Autodesk Inventor part; units mm, degrees
ref_plane "Start plane" through (0, 0, 0) normal (0, 0, 1) x (1, 0, 0)
ref_plane "End plane" through (0, 0, 1500) normal (0, 0, 1) x (1, 0, 0)
ref_plane "YZ Plane" through (0, 0, 0) normal (1, 0, 0) x (0, 1, 0)
ref_plane "Start plane" through (0, 0, 0) normal (0, 0, 1) x (1, 0, 0)
ref_plane "End plane" through (0, 0, 1500) normal (0, 0, 1) x (1, 0, 0)
sketch "Sketch" plane through (0, 0, 0) normal (0, 0, 1) x (1, 0, 0)
  line L0 (-36.5, -70) -> (-36.5, -63.1)
  line L1 (-36.5, -63.1) -> (-9.35, -63.1)
  line L2 (-2.35, -56.1) -> (-2.35, 0)
  line L3 (-2.35, 0) -> (0, 0) construction
  line L4 (0, 0) -> (0, -70) construction
  line L5 (0, -70) -> (-36.5, -70)
  line L6 (-60, 0) -> (80, 0) construction
  line L7 (0, -60) -> (0, 80) construction
  line L8 (36.5, -70) -> (36.5, -63.1)
  line L9 (36.5, -63.1) -> (9.35, -63.1)
  line L10 (2.35, -56.1) -> (2.35, 0)
  line L11 (2.35, 0) -> (0, 0) construction
  line L12 (0, -70) -> (36.5, -70)
  line L13 (-36.5, 70) -> (-36.5, 63.1)
  line L14 (-36.5, 63.1) -> (-9.35, 63.1)
  line L15 (-2.35, 56.1) -> (-2.35, 0)
  line L16 (0, 70) -> (-36.5, 70)
  line L17 (36.5, 70) -> (36.5, 63.1)
  line L18 (36.5, 63.1) -> (9.35, 63.1)
  line L19 (0, 70) -> (36.5, 70)
  line L20 (2.35, 56.1) -> (2.35, 0)
  arc A0 (-2.35, 56.1) -> (-9.35, 63.1) centre (-9.35, 56.1) ccw
  arc A1 (9.35, 63.1) -> (2.35, 56.1) centre (9.35, 56.1) ccw
  arc A2 (2.35, -56.1) -> (9.35, -63.1) centre (9.35, -56.1) ccw
  arc A3 (-9.35, -63.1) -> (-2.35, -56.1) centre (-9.35, -56.1) ccw
  line L21 (0, 108) -> (0, -88) construction
  line L22 (-88, 0) -> (108, 0) construction
  point P0 (-2.35, -63.1)
  point P1 (2.35, -63.1)
  point P2 (-2.35, 63.1)
  point P3 (2.35, 63.1)
  dimension "d1" = 70
  dimension "d2" = 6.9
  dimension "d3" = 36.5
  dimension "d4" = 2.35
  dimension "d10" = 7
extrude "Body" add sketch "Sketch" along normal up to surface (1500 mm away) from surface at 0
sketch "Sketch4" plane through (0, 0, 0) normal (0, 0, 1) x (1, 0, 0)
  line L0 (0, 0) -> (10, 0)
ref_plane "Work Plane3" through (0, 0, 0) normal (0, -1, 0) x (1, 0, 0)
sketch "Sketch5" plane through (0, 0, 0) normal (0, -1, 0) x (1, 0, 0)
  line L0 (-2, 0) -> (12, 0)
  line L1 (-2, 1500) -> (12, 1500)
  dimension "d14" = 1500
equation "\"d1\" = 0.5 * G_H"
equation "\"d2\" = G_T1"
equation "\"d3\" = 0.5 * G_W"
equation "\"d4\" = 0.5 * G_T"
equation "\"d10\" = G_IR"
equation "\"d5\" = G_L"
equation "\"G_W\" = 73"
equation "\"G_T\" = 4.7"
equation "\"G_T1\" = 6.9"
equation "\"G_IR\" = 7"
equation "\"G_L\" = d14"
equation "\"G_OFFSET_START\" = 0"
equation "\"G_OFFSET_END\" = 0"
properties part number "PN-91/H-93419 - IPE140 - 1500" material "Steel, Mild"
Input: part model. Units: mm. Frame: model coordinates. A direction names the side the tool comes from. Coordinates: 2 decimals unless noted, no trailing zeros. Write each loop counter-clockwise with the first axis right and the second up, starting at its lowest first coordinate (ties: lowest second). Pieces come first, ordered by that corner, then holes. Notation, with made-up numbers: M -24.75,56 L -2.75,56 A20 ccw -2.75,80 Z; hole C -36,38 d5. An arc over 180 degrees is marked long. Answer as a JSON object with one key per item and string values. Group by question number.
(1) Ray query, line 1 along Y through (x, z) = (-28, 393); line 2 along X through (y, z) = (-6.5, 1286.5); line 3 along Y through (x, z) = (3, 564). Return the intervals inside material, ascending. Write a range as [from, to].
(2) Contact query for a flat-ended pin moving along its axis: P1, Ø3, axis at y = 23, z = 1046.5, coming from the -X side. Output: stop coordinate, or through.
(3) Set-up query: faces 1 (the face through (1, -70, 740)), 2 (the face through (2.35, 1, 740)), 3 (the face through (-2.35, 1, 740)). Return all of +Z, -Z, +X, -X, +Y, -Y with unobstructed straight access to the full face (end or side cutting, diameter ignored); none if empty.
(4) Section A-A on x = -21. Output: boundary loops of the cut face in (y, z).
(5) Section B-B on z = 730.5. Output: boundary loops of the cut face in (x, y), plus the area to 3 significant figures.
(6) Section C-C on y = -29. Output: boundary loops of the cut face in (x, z), plus the area to 3 significant figures.
Result set:
{
 "1": {"line 1": "y = [-70, -63.1], [63.1, 70]", "line 2": "x = [-2.35, 2.35]", "line 3": "y = [-70, -59.05], [59.05, 70]"},
 "2": {"P1": "stops at x = -2.35"},
 "3": {"face 1": "+Z, -Z, +X, -X, -Y", "face 2": "+Z, -Z, +X", "face 3": "+Z, -Z, -X"},
 "4": {"outline": "M -70,0 L -63.1,0 L -63.1,1500 L -70,1500 Z; M 63.1,0 L 70,0 L 70,1500 L 63.1,1500 Z"},
 "5": {"outline": "M -36.5,-70 L 36.5,-70 L 36.5,-63.1 L 9.35,-63.1 A7 cw 2.35,-56.1 L 2.35,56.1 A7 cw 9.35,63.1 L 36.5,63.1 L 36.5,70 L -36.5,70 L -36.5,63.1 L -9.35,63.1 A7 cw -2.35,56.1 L -2.35,-56.1 A7 cw -9.35,-63.1 L -36.5,-63.1 Z", "area": "1,640 mm2"},
 "6": {"outline": "M -2.35,0 L 2.35,0 L 2.35,1500 L -2.35,1500 Z", "area": "7,050 mm2"}
}
